Design review of the part shown in the three views and the two pictorial views. Dimensions are in mm from the part's minimum x, y and z. Give positions to 0.01 mm unless a question says otherwise; leave off trailing zeros. Order: outer loops, then holes, each group sorted by start corner. A loop starts at its lowest first (then second) coordinate and runs counter-clockwise, first axis right, second up. Notation, with made-up numbers: M -37,27.25 L -27,27.25 A22 cw -27,35.25 Z; hole C 67.25,-5 d8. An arc over 180 degrees is marked long. Answer as a JSON object with one key per item and string values.
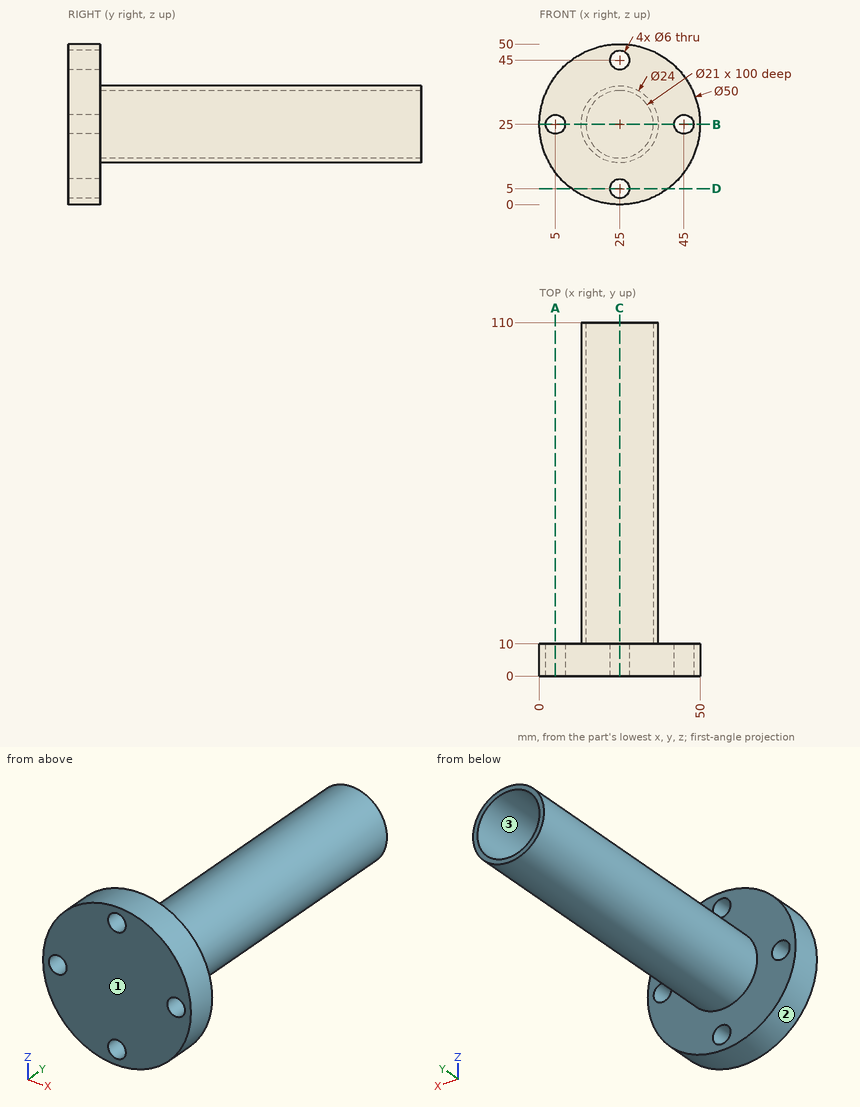
(1) We need section B-B (z = 25). Write out the cut boundary in (x, y).
Checked values:
{"outline": "M 0,0 L 2,0 L 2,10 L 0,10 Z; M 8,0 L 42,0 L 42,10 L 37,10 L 37,110 L 35.5,110 L 35.5,10 L 14.5,10 L 14.5,110 L 13,110 L 13,10 L 8,10 Z; M 48,0 L 50,0 L 50,10 L 48,10 Z"}
(2) To check wall thickness, follow L1, parallel to Z at x = 25, y = 6.5; L2, parallel to X at y = 41, z = 25; L3, parallel to Y at x = 22, z = 42.5. State the ranges of each line that lie inside material, in increasing order. Write a range as from..to.
Checked values:
{"L1": "z = 0..2, 8..42, 48..50", "L2": "x = 13..14.5, 35.5..37", "L3": "y = 0..10"}
(3) We need section C-C (x = 25). Write out the cut boundary in (y, z).
Checked values:
{"outline": "M 0,0 L 10,0 L 10,2 L 0,2 Z; M 0,8 L 10,8 L 10,13 L 110,13 L 110,14.5 L 10,14.5 L 10,35.5 L 110,35.5 L 110,37 L 10,37 L 10,42 L 0,42 Z; M 0,48 L 10,48 L 10,50 L 0,50 Z"}
(4) We need section A-A (x = 5). Write out the cut boundary in (y, z).
Checked values:
{"outline": "M 0,10 L 10,10 L 10,22 L 0,22 Z; M 0,28 L 10,28 L 10,40 L 0,40 Z"}
(5) We need section D-D (z = 5). Write out the cut boundary in (x, y).
Checked values:
{"outline": "M 10,0 L 22,0 L 22,10 L 10,10 Z; M 28,0 L 40,0 L 40,10 L 28,10 Z"}
(6) Insertion check: pin 1 (2 mm diameter, centred on x = 14, z = 38.5, fed in from +Y); pin 2 (9.5 mm diameter, centred on x = 25, z = 5, fed in from -Y); pin 3 (4 mm diameter, centred on x = 23, y = 44.5, fed in from -Z); pin 4 (2 mm diameter, centred on y = 98, z = 35.5, fed in from +X). Each pin has a flat end and moves straight along its axis. Give the tip position at first contact, or say it passes through.
Checked values:
{"pin 1": "stops at y = 10", "pin 2": "stops at y = 0", "pin 3": "stops at z = 13", "pin 4": "stops at x = 32.33"}
(7) Draft analysis for pull direction X (two halves, no side actions). For the marked faces 1, 2 and 3, state which applies: +X half, -X half, draft (parallel to the pull), parting line (faces both ways), or undercut.
Checked values:
{"face 1": "draft", "face 2": "parting line", "face 3": "undercut"}
